from build123d import *

# Parameters (mm, degrees)
SKETCH1_W           = 255
SKETCH1_H           = 120
SKETCH1_R           = 1.6
BASE_FLANGE1_DEPTH  = 5
CUT_EXTRUDE1_REACH  = 143.001
SKETCH9_W           = 5.1
SKETCH9_H           = 30.1
BOSS_EXTRUDE1_DEPTH = 5
SKETCH10_W          = 25
SKETCH10_H          = 15
SKETCH10_W_2        = 10
SKETCH10_H_2        = 5.2
BOSS_EXTRUDE2_DEPTH = 5
FILLET1_R           = 5
FILLET2_R           = 2.5
FILLET3_R           = 10
CUT_EXTRUDE2_DEPTH  = 168.779617356


# Sheet-metal steps are written as plain solids
with BuildPart() as part:
    # Sketch1 → Base-Flange1 (new body)
    with BuildSketch(Plane(origin=(0, 0, 0), x_dir=(1, 0, 0), z_dir=(0, 1, 0))):
        Rectangle(SKETCH1_W, SKETCH1_H)
        with Locations(Location((-112.5, 52.5, 0), (0, 0, 270))):
            Circle(SKETCH1_R, mode=Mode.SUBTRACT)
        with Locations(Location((-112.5, -52.5, 0), (0, 0, 270))):
            Circle(SKETCH1_R, mode=Mode.SUBTRACT)
        with Locations(Location((-7.5, -52.5, 0), (0, 0, 270))):
            Circle(SKETCH1_R, mode=Mode.SUBTRACT)
        with Locations(Location((-7.5, 52.5, 0), (0, 0, 270))):
            Circle(SKETCH1_R, mode=Mode.SUBTRACT)
        with Locations(Location((7.5, 52.5, 0), (0, 0, 270))):
            Circle(SKETCH1_R, mode=Mode.SUBTRACT)
        with Locations(Location((112.5, 52.5, 0), (0, 0, 270))):
            Circle(SKETCH1_R, mode=Mode.SUBTRACT)
        with Locations(Location((112.5, -52.5, 0), (0, 0, 270))):
            Circle(SKETCH1_R, mode=Mode.SUBTRACT)
        with Locations(Location((7.5, -52.5, 0), (0, 0, 270))):
            Circle(SKETCH1_R, mode=Mode.SUBTRACT)
    extrude(amount=-BASE_FLANGE1_DEPTH)

    # Sketch6 → Cut-Extrude1 (cut, up to next)
    with BuildSketch(Plane(origin=(0, 0, 0), x_dir=(1, 0, 0), z_dir=(0, 1, 0)), mode=Mode.PRIVATE) as cut_extrude1_sk1:
        Polygon((-108.125, 56), (-108.125, 47.25), (-116.875, 47.25), (-116.875, -47.25), (-108.125, -47.25), (-108.125, -56), (-13.625, -56), (-13.625, -47.25), (13.625, -47.25), (13.625, -56), (108.125, -56), (108.125, -47.25), (116.875, -47.25), (116.875, 47.25), (108.125, 47.25), (108.125, 56), (13.625, 56), (13.625, 47.25), (-13.625, 47.25), (-13.625, 56), align=None)
    cut_extrude1_tool1 = extrude(cut_extrude1_sk1.sketch, amount=-CUT_EXTRUDE1_REACH, mode=Mode.PRIVATE) & part.part
    add(cut_extrude1_tool1.solids().sort_by_distance((0, 0, 0))[0], mode=Mode.SUBTRACT)

    # Sketch9 → Boss-Extrude1 (add)
    # profile 1 of 2: a face of its own
    with BuildSketch(Plane(origin=(0, 0, 0), x_dir=(1, 0, 0), z_dir=(0, 1, 0))):
        with BuildLine():
            Line((-150, 60), (-150, -31.286796564))
            ThreePointArc((-150, -31.286796564), (-148.858192988, -37.02704805), (-145.606601718, -41.893398282))
            Line((-145.606601718, -41.893398282), (-127.5, -60))
            Line((-127.5, -60), (-127.5, 60))
            Line((-127.5, 60), (-13.625, 60))
            Line((-13.625, 60), (-13.625, 65))
            Line((-13.625, 65), (-150, 65))
            Line((-150, 65), (-150, 60))
        make_face()
        with Locations((-143.45, 35)):
            Rectangle(SKETCH9_W, SKETCH9_H, mode=Mode.SUBTRACT)
    # profile 2 of 2: a face of its own
    with BuildSketch(Plane(origin=(0, 0, 0), x_dir=(1, 0, 0), z_dir=(0, 1, 0))):
        with BuildLine():
            Line((127.5, 60), (127.5, -60))
            Line((127.5, -60), (145, -60))
            ThreePointArc((145, -60), (148.535533906, -58.535533906), (150, -55))
            Line((150, -55), (150, 60))
            Line((150, 60), (150, 65))
            Line((150, 65), (13.625, 65))
            Line((13.625, 65), (13.625, 60))
            Line((13.625, 60), (127.5, 60))
        make_face()
        with Locations((143.45, 35)):
            Rectangle(SKETCH9_W, SKETCH9_H, mode=Mode.SUBTRACT)
    extrude(amount=-BOSS_EXTRUDE1_DEPTH)

    # Sketch10 → Boss-Extrude2 (add)
    # profile 1 of 2: a face of its own
    with BuildSketch(Plane(origin=(0, 0, 0), x_dir=(1, 0, 0), z_dir=(0, 1, 0))):
        with Locations((115, -67.5)):
            Rectangle(SKETCH10_W, SKETCH10_H)
        with Locations((115, -67.5)):
            Rectangle(SKETCH10_W_2, SKETCH10_H_2, mode=Mode.SUBTRACT)
    # profile 2 of 2: a face of its own
    with BuildSketch(Plane(origin=(0, 0, 0), x_dir=(1, 0, 0), z_dir=(0, 1, 0))):
        with Locations((-115, -67.5)):
            Rectangle(SKETCH10_W, SKETCH10_H)
        with Locations((-115, -67.5)):
            Rectangle(SKETCH10_W_2, SKETCH10_H_2, mode=Mode.SUBTRACT)
    extrude(amount=-BOSS_EXTRUDE2_DEPTH)

    # Fillet1
    fillet1_edges = [part.edges().sort_by_distance(p)[0] for p in [
        (102.5, -2.5, 75),
        (127.5, -2.5, 75),
        (-127.5, -2.5, 75),
        (-102.5, -2.5, 75),
    ]]
    fillet(fillet1_edges, radius=FILLET1_R)

    # Fillet2
    fillet2_edges = [part.edges().sort_by_distance(p)[0] for p in [
        (-108.125, -2.5, -56),
        (-13.625, -2.5, -47.25),
        (13.625, -2.5, -47.25),
        (108.125, -2.5, -56),
        (108.125, -2.5, -47.25),
        (116.875, -2.5, -47.25),
        (116.875, -2.5, 47.25),
        (108.125, -2.5, 47.25),
        (108.125, -2.5, 56),
        (13.625, -2.5, 47.25),
        (-13.625, -2.5, 47.25),
        (-108.125, -2.5, 56),
        (-108.125, -2.5, 47.25),
        (-116.875, -2.5, 47.25),
        (-116.875, -2.5, -47.25),
        (-108.125, -2.5, -47.25),
    ]]
    fillet(fillet2_edges, radius=FILLET2_R)

    # Fillet3
    # the kernel refuses this fillet: 10 mm, written as the material it adds along each edge
    with BuildSketch(Plane(origin=(127.5, 0, 60), x_dir=(0, 0, 1), z_dir=(0, -1, 0))) as fillet3_piece_1:
        with BuildLine():
            CenterArc((FILLET3_R, -FILLET3_R), FILLET3_R, 90, 90)
            Line((0, -FILLET3_R), (0, 0))
            Line((0, 0), (FILLET3_R, 0))
        make_face()
    extrude(amount=5)
    with BuildSketch(Plane(origin=(102.5, 0, 60), x_dir=(0, 0, 1), z_dir=(0, -1, 0)), Plane(origin=(-102.5, 0, 60), x_dir=(1, 0, 0), z_dir=(0, -1, 0))) as fillet3_piece_2:
        with BuildLine():
            CenterArc((FILLET3_R, FILLET3_R), FILLET3_R, 180, 90)
            Line((0, FILLET3_R), (0, 0))
            Line((0, 0), (FILLET3_R, 0))
        make_face()
    extrude(amount=5)
    with BuildSketch(Plane(origin=(-13.625, 0, -56), x_dir=(-1, 0, 0), z_dir=(0, -1, 0))) as fillet3_piece_3:
        with BuildLine():
            CenterArc((9.424240018, -10), FILLET3_R, 90, 72.542396876)
            Line((-0.115151996, -7), (-1.069091198, -6.7))
            ThreePointArc((-1.069091198, -6.7), (-1, -6.25), (-1, 0))
            Line((-1, 0), (0, 1))
            Line((0, 1), (9.424240018, 1))
            Line((9.424240018, 1), (9.424240018, 0))
        make_face()
    extrude(amount=5)
    with BuildSketch(Plane(origin=(13.625, 0, -56), x_dir=(-0.01644805983855046, 0, 0.9998647215136394), z_dir=(0, -1, 0))) as fillet3_piece_4:
        with BuildLine():
            CenterArc((9.843636751, -9.587445719), FILLET3_R, 106.515156216, 72.542396876)
            Line((-0.155010464, -9.422965121), (-1.154875185, -9.406517061))
            Line((-1.154875185, -9.406517061), (-0.999864722, 0.01644806))
            Line((-0.999864722, 0.01644806), (0.01644806, 0.999864722))
            ThreePointArc((0.01644806, 0.999864722), (6.265602569, 0.897064348), (6.71667811, 0.958744572))
            Line((6.71667811, 0.958744572), (7.000947078, 0))
        make_face()
    extrude(amount=5)
    with BuildSketch(Plane(origin=(13.625, 0, 56), x_dir=(-0.01644805983855046, 0, -0.9998647215136394), z_dir=(0, -1, 0))) as fillet3_piece_5:
        with BuildLine():
            CenterArc((9.843636751, 9.587445719), FILLET3_R, 180.942446908, 72.542396876)
            Line((-0.155010464, 9.422965121), (-1.154875185, 9.406517061))
            Line((-1.154875185, 9.406517061), (-0.999864722, -0.01644806))
            Line((-0.999864722, -0.01644806), (0.01644806, -0.999864722))
            ThreePointArc((0.01644806, -0.999864722), (6.265602569, -0.897064348), (6.71667811, -0.958744572))
            Line((6.71667811, -0.958744572), (7.000947078, 0))
        make_face()
    extrude(amount=5)
    with BuildSketch(Plane(origin=(-13.625, 0, 56), x_dir=(-1, 0, 0), z_dir=(0, -1, 0))) as fillet3_piece_6:
        with BuildLine():
            CenterArc((9.424240018, 10), FILLET3_R, 197.457603124, 72.542396876)
            Line((-0.115151996, 7), (-1.069091198, 6.7))
            ThreePointArc((-1.069091198, 6.7), (-1, 6.25), (-1, 0))
            Line((-1, 0), (0, -1))
            Line((0, -1), (9.424240018, -1))
            Line((9.424240018, -1), (9.424240018, 0))
        make_face()
    extrude(amount=5)
    with BuildSketch(Plane(origin=(-127.5, 0, 60), x_dir=(0, 0, 1), z_dir=(0, -1, 0))) as fillet3_piece_7:
        with BuildLine():
            CenterArc((FILLET3_R * 0.414213562373, FILLET3_R), FILLET3_R, 225, 45)
            Line((-FILLET3_R * 0.292893218813, FILLET3_R * 0.292893218813), (0, 0))
            Line((0, 0), (FILLET3_R * 0.414213562373, 0))
        make_face()
    extrude(amount=5)

    # Sketch11 → Cut-Extrude2 (cut, through all)
    with BuildSketch(Plane(origin=(0, 0, 0), x_dir=(1, 0, 0), z_dir=(0, 1, 0))):
        with BuildLine():
            Line((116.875, 49.75), (116.875, 53.5))
            ThreePointArc((116.875, 53.5), (117.607233047, 55.267766953), (119.375, 56))
            Line((119.375, 56), (134.375, 56))
            ThreePointArc((134.375, 56), (136.142766953, 55.267766953), (136.875, 53.5))
            Line((136.875, 53.5), (136.875, -53.5))
            ThreePointArc((136.875, -53.5), (136.142766953, -55.267766953), (134.375, -56))
            Line((134.375, -56), (119.375, -56))
            ThreePointArc((119.375, -56), (117.607233047, -55.267766953), (116.875, -53.5))
            Line((116.875, -53.5), (116.875, -49.75))
            ThreePointArc((116.875, -49.75), (116.142766953, -47.982233047), (114.375, -47.25))
            ThreePointArc((114.375, -47.25), (116.142766953, -46.517766953), (116.875, -44.75))
            Line((116.875, -44.75), (116.875, 44.75))
            ThreePointArc((116.875, 44.75), (116.142766953, 46.517766953), (114.375, 47.25))
            ThreePointArc((114.375, 47.25), (116.142766953, 47.982233047), (116.875, 49.75))
        make_face()
    extrude(amount=-CUT_EXTRUDE2_DEPTH, mode=Mode.SUBTRACT)


solid = part.part
Model file for the job. Use its own axes, mm. A direction names the side the tool comes from. Coordinates: 2 decimals unless noted, no trailing zeros. Order: outer loops, then holes, each group sorted by start corner. A loop starts at its lowest first (then second) coordinate and runs counter-clockwise, first axis right, second up. Notation, with made-up numbers: (60.5, 5) -> (84.5, 5) arc R25 ccw to (84.5, 37) -> close; hole circle Ø2 at (43.5, 12.25). An arc over 180 degrees is marked (long way). Return JSON: item names as keys, results as strings. Group by question number.
Item 1: Saw through at B-B on z = 35.5. Write the cut outline in (x, y) (3 decimals), then the cut area to 3 significant figures.
Item 2: Pull direction Z, two halves, no side cores. Call faces 4 (the flat face through (-81, -2, -65)), 5 (the flat face through (-1, -2, 60)), 6 (the cylindrical face through (17.06, -2.46, -54.01)): pulls with the +Z half, pulls with the -Z half, needs draft (parallel to the pull), parting line crosses it, or undercut.
Item 3: Flat gauge pins, fed straight in: P1, Ø2.5, axis at x = -5.5, y = -3.5, coming from the +Z side; P2, Ø5, axis at x = 112.5, z = -52.5, coming from the +Y side; P3, Ø2.5, axis at x = 129.5, y = -3, coming from the +Z side. Where does each tip first touch, or does it go through?
Item 4: Wall check: line 1 along Z through (x, y) = (112.5, -3.1); line 2 along X through (y, z) = (-4.6, 5) (3 decimals); line 3 along Z through (x, y) = (64, -2.55). Give the ranges that are in metal, low to high. Write a range as [from, to].
Item 5: Saw through at A-A on x = -82. Write the cut outline in (y, z), then the cut area to 3 significant figures.
Item 6: Saw through at C-C on y = -2.5. State how many separate pieces and enclosed holes the cut face has, then the cut area to 3 significant figures.
Item 7: Tool access for faces 1 (the flat face through (83, -2, -65)), 2 (the flat face through (127, -2, 56)), 3 (the cylindrical face through (99.49, -2.46, 62.85)): list every direction of +Z, -Z, +X, -X, +Y, -Y with a clear straight run to the whole face (end or side of a thin tool).
Values found:
{
 "1": {"outline": "(-149.396, -5) -> (-116.875, -5) -> (-116.875, 0) -> (-149.396, 0) -> close; (136.875, -5) -> (150, -5) -> (150, 0) -> (136.875, 0) -> close", "area": "228 mm2"},
 "2": {"face 4": "pulls with the -Z half", "face 5": "pulls with the +Z half", "face 6": "undercut"},
 "3": {"P1": "stops at z = 60", "P2": "stops at y = 0", "P3": "stops at z = 66.2"},
 "4": {"line 1": "z = [-65, -54.1], [-50.9, -47.25], [47.25, 50.9], [54.1, 64.9], [70.1, 75]", "line 2": "x = [-150, -116.875], [136.875, 150]", "line 3": "z = [-65, -56], [56, 60]"},
 "5": {"outline": "(-5, -65) -> (0, -65) -> (0, -56) -> (-5, -56) -> close; (-5, 56) -> (0, 56) -> (0, 60) -> (-5, 60) -> close", "area": "65.0 mm2"},
 "6": {"separate pieces": "1", "enclosed holes": "13", "area": "9,850 mm2"},
 "7": {"face 1": "-Z, +X, -X, +Y, -Y", "face 2": "+Y, -Y", "face 3": "+Z, +Y, -Y"}
}
